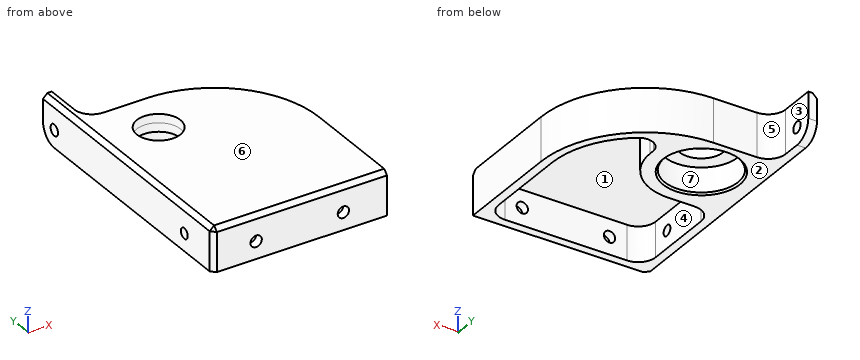
```python
from build123d import *

# Parameters (mm, degrees)
F0_R      = 21
F0_R_2    = 12.5
F1_DEPTH  = 5
F2_DEPTH  = 20
F3_W      = 5
F3_H      = 25
F4_DEPTH  = 30
F6_R      = 3.25
F7_DEPTH  = 25
F5_R      = 3
F5_R_2    = 3.25
F8_DEPTH  = 25
F9_SIZE   = 2.5
F10_R     = 10
F11_DEPTH = 5
F12_SIZE  = 1


# Not quite as in the source:
# - a feature names something its author has since deleted; it is built from what else it names


with BuildPart() as f1:
    # F0 (on Top) → F1 (new body)
    with BuildSketch(Plane.XY):
        with BuildLine():
            Line((30, 65), (5, 65))
            Line((5, 65), (5, 5))
            Line((5, 5), (95, 5))
            Line((95, 5), (95, 61.8416720113))
            ThreePointArc((95, 61.8416720113), (89.0121465356, 85.9307991151), (72.4423646792, 104.4127568838))
            ThreePointArc((72.4423646792, 104.4127568838), (64.4445964825, 104.6534027902), (60, 98))
            Line((60, 98), (60, 95))
            ThreePointArc((60, 95), (51.2132034356, 73.7867965644), (30, 65))
        make_face()
        with BuildLine():
            Line((40, 120), (5, 120))
            Line((5, 120), (5, 65))
            Line((5, 65), (30, 65))
            ThreePointArc((30, 65), (51.2132034356, 73.7867965644), (60, 95))
            Line((60, 95), (60, 98))
            ThreePointArc((60, 98), (64.4445964825, 104.6534027902), (72.4423646792, 104.4127568838))
            ThreePointArc((72.4423646792, 104.4127568838), (89.0121465356, 85.9307991151), (95, 61.8416720113))
            Line((95, 61.8416720113), (95, 5))
            Line((95, 5), (100, 5))
            Line((100, 5), (100, 60))
            ThreePointArc((100, 60), (82.4264068712, 102.4264068712), (40, 120))
        make_face()
        with Locations((30, 94)):
            Circle(F0_R, mode=Mode.SUBTRACT)
        with Locations((30, 94)):
            Circle(F0_R)
        with Locations((30, 94)):
            Circle(F0_R_2, mode=Mode.SUBTRACT)
        Polygon((0, 120), (0, 0), (100, 0), (100, 5), (95, 5), (5, 5), (5, 65), (5, 120), align=None)
    extrude(amount=F1_DEPTH)

    # F0 (on Top) → F2 (join)
    with BuildSketch(Plane.XY):
        Polygon((0, 120), (0, 0), (100, 0), (100, 5), (95, 5), (5, 5), (5, 65), (5, 120), align=None)
        with BuildLine():
            Line((40, 120), (5, 120))
            Line((5, 120), (5, 65))
            Line((5, 65), (30, 65))
            ThreePointArc((30, 65), (51.2132034356, 73.7867965644), (60, 95))
            Line((60, 95), (60, 98))
            ThreePointArc((60, 98), (64.4445964825, 104.6534027902), (72.4423646792, 104.4127568838))
            ThreePointArc((72.4423646792, 104.4127568838), (89.0121465356, 85.9307991151), (95, 61.8416720113))
            Line((95, 61.8416720113), (95, 5))
            Line((95, 5), (100, 5))
            Line((100, 5), (100, 60))
            ThreePointArc((100, 60), (82.4264068712, 102.4264068712), (40, 120))
        make_face()
        with Locations((30, 94)):
            Circle(F0_R, mode=Mode.SUBTRACT)
    extrude(amount=-F2_DEPTH)

    # F3 (on face) → F4 (join)
    with BuildSketch(Plane(origin=(0, 120, 0), x_dir=(-1, 0, 0), z_dir=(0, 1, 0))):
        with Locations((-2.5, -7.5)):
            Rectangle(F3_W, F3_H)
    extrude(amount=F4_DEPTH)

    # F6 (on face) → F7 (cut)
    with BuildSketch(Plane.XZ):
        with Locations((25, -10)):
            Circle(F6_R)
        with Locations((75, -10)):
            Circle(F6_R)
    extrude(amount=-F7_DEPTH, mode=Mode.SUBTRACT)

    # F5 (on face) → F8 (cut)
    with BuildSketch(Plane(origin=(0, 0, 0), x_dir=(0, -1, 0), z_dir=(-1, 0, 0))):
        with Locations((-25, -10)):
            Circle(F5_R)
        with Locations((-140, -10)):
            Circle(F5_R_2)
    extrude(amount=-F8_DEPTH, mode=Mode.SUBTRACT)

    # F9
    f9_edges = [f1.edges().sort_by_distance(p)[0] for p in [
        (50, 0, 5),
        (0, 75, 5),
        (0, 0, -7.5),
    ]]
    chamfer(f9_edges, length=F9_SIZE)

    # F10
    f10_edges = [f1.edges().sort_by_distance(p)[0] for p in [
        (5, 5, -10),
        (95, 5, -10),
        (5, 65, -10),
        (5, 120, -7.5),
        (2.5, 150, -20),
    ]]
    fillet(f10_edges, radius=F10_R)

    # F0 (on Top) → F11 (join)
    with BuildSketch(Plane.XY):
        with Locations((30, 94)):
            Circle(F0_R)
        with Locations((30, 94)):
            Circle(F0_R_2, mode=Mode.SUBTRACT)
    extrude(amount=-F11_DEPTH)

    # F12
    f12_edges = [f1.edges().sort_by_distance(p)[0] for p in [
        (9, 94, -20),
    ]]
    chamfer(f12_edges, length=F12_SIZE)


solid = f1.part
```
Verification items for the finished model (mm, model axes). Face numbers are marked on the shaded views. A direction names the side the tool comes from. Coordinates: 2 decimals unless noted, no trailing zeros. Write each loop counter-clockwise with the first axis right and the second up, starting at its lowest first coordinate (ties: lowest second). Pieces come first, ordered by that corner, then holes. Notation, with made-up numbers: M 62,66 L 86,66 A26 ccw 86,94 Z; hole C -4,33.5 d9. An arc over 180 degrees is marked long. Answer as a JSON object with one key per item and string values. Group by question number.
(1) Gauge pin test, flat ends, axial feed: pin 1 (4 mm diameter, centred on x = 31.5, z = -7.5, fed in from +Y); pin 2 (0.9 mm diameter, centred on y = 97, z = -11, fed in from +X); pin 3 (3 mm diameter, centred on x = 40, y = 62.5, fed in from -Z). Record the tip position at first contact, or that the pin passes through.
(2) Cross-section at B-B, the plane z = -3.25. Record the cut outline in (x, y), and give its area (3 significant figures).
(3) Tool access check on the marked faces 1, 2 and 3. Record the directions out of +Z, -Z, +X, -X, +Y, -Y that give a thin tool (end or side, any length) a straight path to the whole face; none if there is none.
(4) Cross-section at D-D, the plane x = 63.5. Record the cut outline in (y, z).
(5) Cross-section at A-A, the plane y = 25. Record the cut outline in (x, z), and give its area (3 significant figures).
(6) Cross-section at C-C, the plane x = 75. Record the cut outline in (y, z), and give its area (3 significant figures).
(7) Material ranges on line 1 (Y direction, x = 30, z = -9); line 2 (X direction, y = 35, z = -10.5); line 3 (Z direction, x = 47, y = 38.5), recorded low to high.
(8) Release check for a two-part mould opening along Y. For the marked faces 4, 5, 6 and 7 record: +Y half, -Y half, draft (parallel to the pull), parting line (faces both ways), or undercut.
Reply:
{
 "1": {"pin 1": "y = 120", "pin 2": "x = 87.58", "pin 3": "z = 0"},
 "2": {"outline": "M 0,2.5 L 2.5,0 L 100,0 L 100,60 A60 ccw 40,120 L 15,120 A10 cw 5,130 L 5,150 L 0,150 Z; hole M 5,15 A10 ccw 15,5 L 85,5 A10 ccw 95,15 L 95,61.84 A51.45 ccw 72.44,104.41 A8.25 ccw 60,98 L 60,95 A30 cw 30,65 L 15,65 A10 ccw 5,55 Z; hole C 30,94 d25", "area": "4,280 mm²"},
 "3": {"face 1": "-Z", "face 2": "-Z, +X, -X, +Y, -Y", "face 3": "+Z, -Z, +X, +Y"},
 "4": {"outline": "M 0,-20 L 5,-20 L 5,0 L 104.08,0 L 104.08,-20 L 115.21,-20 L 115.21,5 L 2.5,5 L 0,2.5 Z"},
 "5": {"outline": "M 0,-20 L 5,-20 L 5,-13 L 0,-13 Z; M 0,-7 L 5,-7 L 5,0 L 95,0 L 95,-20 L 100,-20 L 100,5 L 2.5,5 L 0,2.5 Z", "area": "667 mm²"},
 "6": {"outline": "M 0,-20 L 5,-20 L 5,-13.25 L 0,-13.25 Z; M 0,-6.75 L 5,-6.75 L 5,0 L 102.56,0 L 102.56,-20 L 108.73,-20 L 108.73,5 L 2.5,5 L 0,2.5 Z", "area": "732 mm²"},
 "7": {"line 1": "0 to 5, 65 to 73, 115 to 120", "line 2": "0 to 5, 95 to 100", "line 3": "0 to 5"},
 "8": {"face 4": "undercut", "face 5": "+Y half", "face 6": "draft", "face 7": "undercut"}
}
